```python
from build123d import *

# Parameters (mm, degrees)
SKETCH_1_R      = 6.5
SKETCH_1_R_2    = 2
EXTRUDE_1_DEPTH = 2.5
CHAMFER_1_SIZE  = 0.1


with BuildPart() as part:
    # 草图1 → 凸台-拉伸1 (new body, symmetric)
    with BuildSketch(Plane.XY):
        Circle(SKETCH_1_R)
        Circle(SKETCH_1_R_2, mode=Mode.SUBTRACT)
    extrude(amount=EXTRUDE_1_DEPTH, both=True)

    # 倒角1
    chamfer_1_edges = [part.edges().sort_by_distance(p)[0] for p in [
        (-6.5, 0, -2.5),
        (-6.5, 0, 2.5),
        (-2, 0, -2.5),
        (-2, 0, 2.5),
    ]]
    chamfer(chamfer_1_edges, length=CHAMFER_1_SIZE)


solid = part.part
```
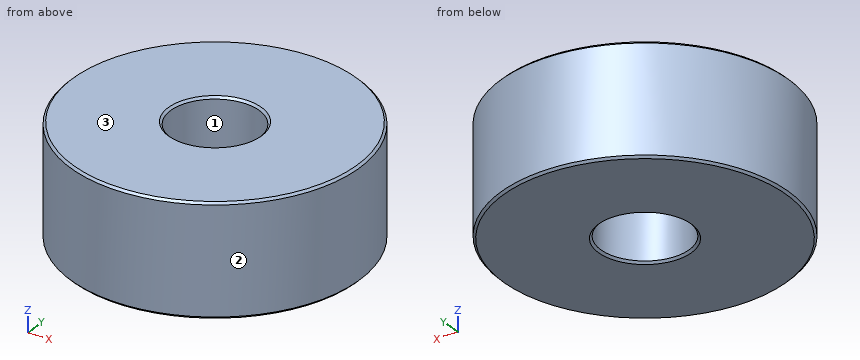
Here's how the part is built. I have some questions about the finished solid (model axes, mm). Face numbers are marked on the shaded views. Give positions to 0.01 mm unless a question says otherwise; leave off trailing zeros. Loops run counter-clockwise (first coordinate to the right, second up) from the corner with the lowest first, then second, coordinate; pieces in that order, holes last. Notation, with made-up numbers: M 10,7.5 L 53,7.5 A20 cw 53,20.5 Z; hole C -26,33 d4. An arc over 180 degrees is marked long. Return JSON: item names as keys, results as strings.
Item 1: Imagine slicing it at C-C on z = -0.65. List the corners of the cut face in (x, y) for me.
A:
{"outline": "C 0,0 d13; hole C 0,0 d4"}
Item 2: Thinking about a two-plate mould opening in Y: for the marked faces 1, 2 and 3, which applies, released by +Y, released by -Y, zero draft, split by the parting line, or undercut?
A:
{"face 1": "undercut", "face 2": "split by the parting line", "face 3": "zero draft"}
Item 3: I'm going to push a flat-ended pin straight in: pin 1 Ø2 at (y, z) = (2.5, 0) entering from -X. Where does the tip first touch, or does it pass through?
A:
{"pin 1": "stops at x = -6.32"}
Item 4: Please list where these lines run through material, in increasing order: line 1 (Y direction, x = 0, z = -0.4); line 2 (Y direction, x = -1.25, z = -1.4); line 3 (X direction, y = -1.5, z = -1.3).
A:
{"line 1": "y = -6.5 to -2, 2 to 6.5", "line 2": "y = -6.38 to -1.56, 1.56 to 6.38", "line 3": "x = -6.32 to -1.32, 1.32 to 6.32"}
Item 5: Imagine slicing it at A-A on x = 0. List the corners of the cut face in (y, z) for me, then the cut area to 3 significant figures.
A:
{"outline": "M -6.5,-2.4 L -6.4,-2.5 L -2.1,-2.5 L -2,-2.4 L -2,2.4 L -2.1,2.5 L -6.4,2.5 L -6.5,2.4 Z; M 2,-2.4 L 2.1,-2.5 L 6.4,-2.5 L 6.5,-2.4 L 6.5,2.4 L 6.4,2.5 L 2.1,2.5 L 2,2.4 Z", "area": "45.0 mm^2"}
